The model under review builds one solid part; all positions refer to its coordinate system, in mm. Face numbers are marked on the shaded views. A direction names the side the tool comes from. Coordinates: 2 decimals unless noted, no trailing zeros. Order: outer loops, then holes, each group sorted by start corner. A loop starts at its lowest first (then second) coordinate and runs counter-clockwise, first axis right, second up. Notation, with made-up numbers: M -34,67.25 L 15,67.25 A27 ccw 15,94.25 Z; hole C 15.25,-34 d1. An arc over 180 degrees is marked long. Answer in a Markdown table with one row per item.
from build123d import *


with BuildPart() as part:
    # Croquis1 → Revolución1 (revolve)
    with BuildSketch(Plane.XY, mode=Mode.PRIVATE) as revoluci_n1_sk:
        with BuildLine():
            Line((-23, 68), (-18, 68))
            Line((-18, 68), (-18, 63))
            Line((-18, 63), (18, 63))
            Line((18, 63), (18, 68))
            Line((18, 68), (23, 68))
            Line((23, 68), (23, 63))
            Line((23, 63), (33, 53))
            Line((33, 53), (33, 51))
            Line((33, 51), (27, 30))
            ThreePointArc((27, 30), (31.485292704, 15.297058541), (33, 0))
            Line((33, 0), (-23, 0))
            Line((-23, 0), (-23, 8))
            Line((-23, 8), (-29, 8))
            Line((-29, 8), (-29, 16.5))
            Line((-29, 16.5), (-23, 22.5))
            Line((-23, 22.5), (-23, 68))
        make_face()
    revolve(revoluci_n1_sk.sketch.rotate(Axis((-754.889867841, 0, 0), (1, 0, 0)), 90), axis=Axis((-754.889867841, 0, 0), (1, 0, 0)))


solid = part.part
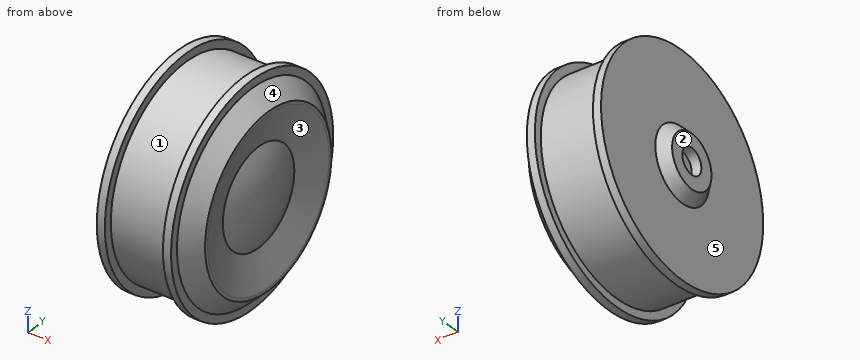
(1) To check wall thickness, follow line 1 (X direction, y = 59, z = 23); line 2 (Y direction, x = -25, z = 0); line 3 (Y direction, x = 9, z = 0). State the ranges of each line that lie inside material, in increasing order. Write a range as [from, to].
Report:
| item | result |
|---|---|
| line 1 | [-23, -18], [18, 23] |
| line 2 | [-20.5, -8], [8, 20.5] |
| line 3 | [-63, 63] |
(2) The part is to be moulded in two halves that separate along Y. For the marked faces 3, 4 and 5, say which applies: +Y half, -Y half, draft (parallel to the pull), parting line (faces both ways), or undercut.
Report:
| item | result |
|---|---|
| face 3 | undercut |
| face 4 | parting line |
| face 5 | draft |
(3) Machinability: for the marked faces 1 and 2, which of the approach directions +Z, -Z, +X, -X, +Y, -Y give a long, thin tool a straight path to every point of the face, cutting with its end or side? Answer none if there is none.
Report:
| item | result |
|---|---|
| face 1 | none |
| face 2 | +Z, -Z, -X, +Y, -Y |
(4) Insertion check: P1, Ø12, axis at x = 19, z = -54.5, coming from the +Y side; P2, Ø2, axis at y = -29.5, z = 31, coming from the -X side; P3, Ø4, axis at x = -7, y = -16, coming from the -Z side. Each pin has a flat end and moves straight along its axis. Give the tip position at first contact, or say it passes through.
Report:
| item | result |
|---|---|
| P1 | y = 47.66 |
| P2 | x = -23 |
| P3 | z = -61.42 |
(5) Take a section at C-C (x = 0.5). Write out the cut boundary in (y, z).
Report:
| item | result |
|---|---|
| outline | C 0,0 d126 |
(6) Take a section at A-A (z = 0). Write out the cut boundary in (x, y), then the cut area to 3 significant figures.
Report:
| item | result |
|---|---|
| outline | M -29,-16.5 L -23,-22.5 L -23,-68 L -18,-68 L -18,-63 L 18,-63 L 18,-68 L 23,-68 L 23,-63 L 33,-53 L 33,-51 L 27,-30 A78 ccw 27,30 L 33,51 L 33,53 L 23,63 L 23,68 L 18,68 L 18,63 L -18,63 L -18,68 L -23,68 L -23,22.5 L -29,16.5 L -29,8 L -23,8 L -23,-8 L -29,-8 Z |
| area | 6,950 mm^2 |
